Here's the drawing with two shaded views (mm, measured from the low corner). I have some questions. Give positions to 0.01 mm unless a question says otherwise; leave off trailing zeros. Loops run counter-clockwise (first coordinate to the right, second up) from the corner with the lowest first, then second, coordinate; pieces in that order, holes last. Notation, with made-up numbers: M 0,37.25 L 36,37.25 A29 cw 36,76.25 Z; hole C 71,-29 d3. An arc over 180 degrees is marked long. Answer in a Markdown table with one row per item. Add a question column.
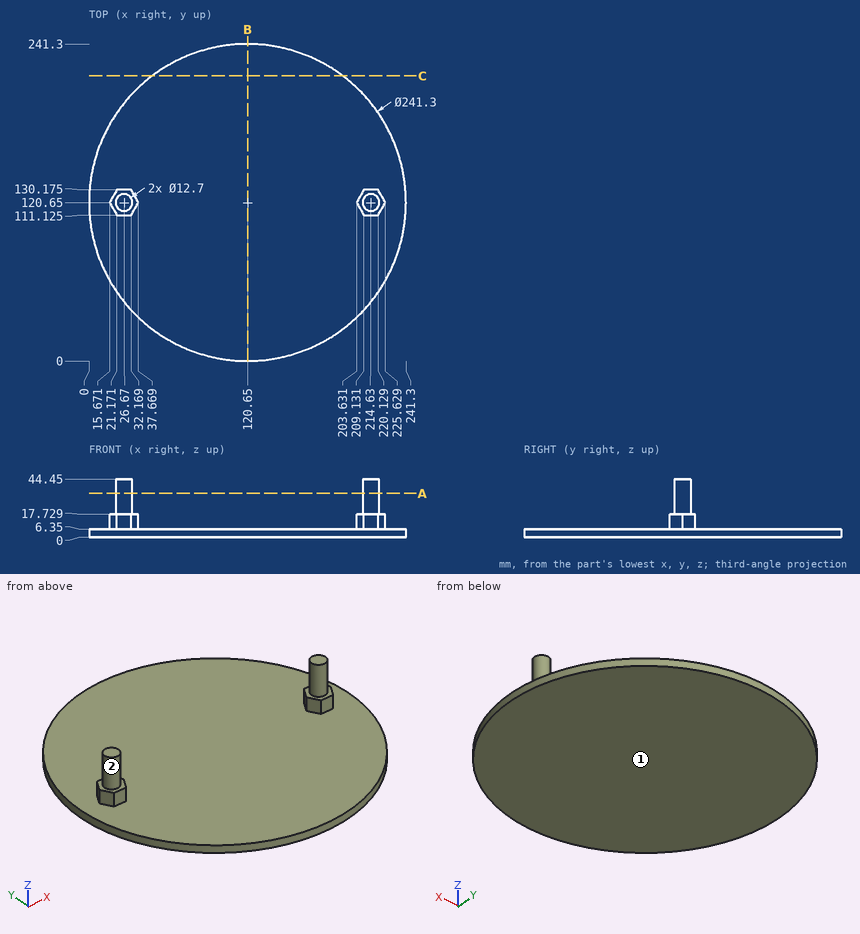
Item 1: If we mould it in two halves opening along X, with no side actions, what happens to the marked faces 1 and 2? For each: +X half, -X half, draft (parallel to the pull), parting line (faces both ways), or undercut.
Item 2: I need wall thicknesses on L1, parallel to Z at x = 126, y = 151; L2, parallel to Y at x = 214.5, z = 21.5; L3, parallel to X at y = 128.5, z = 16 (1 decimal). Which ranges of each line are inside material? Lowest first, please.
Item 3: Suppose I cut it at B-B (x = 120.65). List the corners of the cut face in (y, z) for me.
Item 4: Suppose I cut it at C-C (y = 217). List the corners of the cut face in (x, z) for me.
Item 5: For P1, Ø3.5, axis at x = 26, z = 10.5, coming from the -Y side (3 decimals); P2, Ø4, axis at x = 164, y = 181, coming from the -Z side; P3, Ø2, axis at x = 114, y = 155, coming from the +Z side; P4, Ø5.5, axis at x = 217, z = 14, coming from the +Y side (3 decimals), each with a flat end and sliding along its axis, tell me the tip position at first contact or that it passes through.
Item 6: Suppose I cut it at A-A (z = 33.5). List the corners of the cut face in (x, y) for me, then the cut area to 3 significant figures.
Values found:
| question | item | result |
|---|---|---|
| 1 | face 1 | draft |
| 1 | face 2 | undercut |
| 2 | L1 | 0 to 6.35 |
| 2 | L2 | 114.3 to 127 |
| 2 | L3 | 20.2 to 33.1, 208.2 to 221.1 |
| 3 | outline | M 0,0 L 241.3,0 L 241.3,6.35 L 0,6.35 Z |
| 4 | outline | M 48.03,0 L 193.27,0 L 193.27,6.35 L 48.03,6.35 Z |
| 5 | P1 | y = 111.125 |
| 5 | P2 | z = 0 |
| 5 | P3 | z = 6.35 |
| 5 | P4 | y = 130.175 |
| 6 | outline | C 26.67,120.65 d12.7; C 214.63,120.65 d12.7 |
| 6 | area | 253 mm² |
